For this review, take the finished solid that the model builds, in its own axes (mm). Face numbers are marked on the shaded views. A direction names the side the tool comes from. Round coordinates to 2 decimals unless told otherwise and drop trailing zeros. Loops run counter-clockwise (first coordinate to the right, second up) from the corner with the lowest first, then second, coordinate; pieces in that order, holes last.
1. To check wall thickness, follow line 1 along Z through (x, y) = (26.4, 15.24); line 2 along Z through (x, y) = (24.75, 15.5); line 3 along X through (y, z) = (25.5, -4) (3 decimals). State the ranges of each line that lie inside material, in increasing order.
2. Consider section B-B on z = -56. State the section outline as (x, y) points (3 decimals).
3. Tool access review of the marked faces 4, 5 and 6: name each direction out of +Z, -Z, +X, -X, +Y, -Y from which nothing blocks a thin tool from reaching the whole face with its end or side.
4. Consider section A-A on y = 15.24. State how many separate pieces and enclosed holes the cut face has, then the cut area to 3 significant figures.
5. Consider section D-D on z = -31.75. State the section outline as (x, y) points.
6. Clearance check with flat-ended pins moving along their axes: pin 1 Ø3 at (y, z) = (15.24, -56.42) entering from +X; pin 2 Ø3.5 at (y, z) = (12.5, -59) entering from -X; pin 3 Ø1 at (x, y) = (20.5, 20.5) entering from +Z; pin 4 Ø1.5 at (y, z) = (12.5, -16) entering from +X. State where each tip first meets the part, or that it passes through.
7. Consider section C-C on y = 18.25. State the section outline as (x, z) points (3 decimals).
8. Draft analysis for pull direction Z (two halves, no side actions). For the marked faces 1, 2 and 3, state which applies: released by +Z, released by -Z, zero draft, split by the parting line, or undercut.
from build123d import *

# Parameters (mm, degrees)
BOSS_EXTRUDE14_DEPTH = 2.54
BOSS_EXTRUDE15_DEPTH = 26.67
SKETCH5_R            = 1.905
CUT_EXTRUDE12_DEPTH  = 29.575
FILLET3_R            = 2.54


with BuildPart() as part:
    # Sketch3 → Boss-Extrude14 (new body)
    with BuildSketch(Plane(origin=(0, 0, 0), x_dir=(1, 0, 0), z_dir=(0, 1, 0))):
        with BuildLine():
            Line((0, 63.5), (0, 0))
            Line((0, 0), (24.257, 0))
            Line((24.257, 0), (24.257, 10.953386454))
            ThreePointArc((24.257, 10.953386454), (7.334843244, 31.75), (24.257, 52.546613546))
            Line((24.257, 52.546613546), (24.257, 63.5))
            Line((24.257, 63.5), (0, 63.5))
        make_face()
    extrude(amount=BOSS_EXTRUDE14_DEPTH)

    # Sketch3<18> → Boss-Extrude15 (add)
    with BuildSketch(Plane(origin=(0, 0, 0), x_dir=(1, 0, 0), z_dir=(0, 1, 0))):
        with BuildLine():
            Line((24.257, 10.953386454), (24.257, 0))
            Line((24.257, 0), (28.575, 0))
            Line((28.575, 0), (28.575, 13.081))
            ThreePointArc((28.575, 13.081), (9.906, 31.75), (28.575, 50.419))
            Line((28.575, 50.419), (28.575, 63.5))
            Line((28.575, 63.5), (24.257, 63.5))
            Line((24.257, 63.5), (24.257, 52.546613546))
            ThreePointArc((24.257, 52.546613546), (7.334843244, 31.75), (24.257, 10.953386454))
        make_face()
    extrude(amount=BOSS_EXTRUDE15_DEPTH)

    # Sketch5 → Cut-Extrude12 (cut, through all)
    with BuildSketch(Plane(origin=(0, 0, 0), x_dir=(0, 0, -1), z_dir=(1, 0, 0))):
        with Locations((6.5405, 15.24)):
            Circle(SKETCH5_R)
        with Locations((56.41762459, 15.24)):
            Circle(SKETCH5_R)
    extrude(amount=CUT_EXTRUDE12_DEPTH, mode=Mode.SUBTRACT)

    # Fillet3
    fillet3_edges = [part.edges().sort_by_distance(p)[0] for p in [
        (24.257, 2.54, -58.023306773),
        (24.257, 2.54, -5.476693227),
        (7.334843244, 2.54, -31.75),
    ]]
    fillet(fillet3_edges, radius=FILLET3_R)


solid = part.part
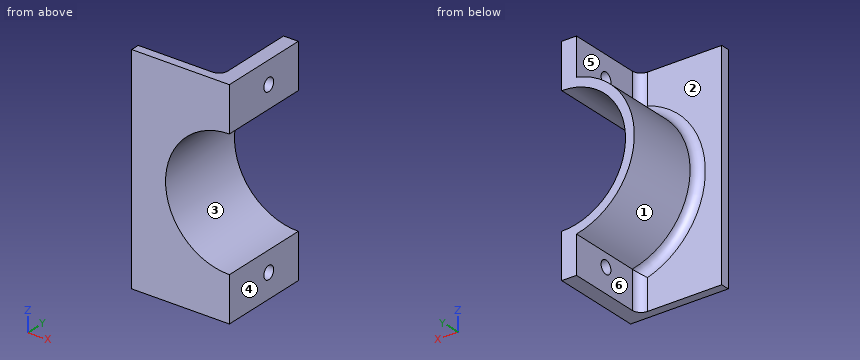
Resolved:
1. line 1: z = -63.5 to -58.32, -54.51 to -50.29, -13.21 to -8.45, -4.64 to 0
1. line 2: z = -63.5 to -58.3, -54.53 to -50.02, -13.48 to -8.43, -4.65 to 0
1. line 3: x = 24.257 to 28.575
2. outline: (0, 0) - (28.575, 0) - (28.575, 13.381) - (24.257, 13.381) - (24.257, 5.08) arc R2.54 cw to (21.717, 2.54) - (0, 2.54) - close; (24.257, 17.099) - (28.575, 17.099) - (28.575, 26.67) - (24.257, 26.67) - close
3. face 4: +Z, -Z, +X, +Y, -Y
3. face 5: +Z, -X, +Y
3. face 6: -Z, -X, +Y
4. separate pieces: 3
4. enclosed holes: 0
4. area: 220 mm2
5. outline: (0, 0) - (9.91, 0) - (9.91, 26.67) - (7.33, 26.67) - (7.33, 5.08) arc R2.54 cw to (4.79, 2.54) - (0, 2.54) - close
6. pin 1: passes through
6. pin 2: stops at x = 24.26
6. pin 3: stops at z = -11.91
6. pin 4: stops at x = 19.84
7. outline: (24.257, -63.5) - (28.575, -63.5) - (28.575, -50.419) arc R18.669 cw to (28.575, -13.081) - (28.575, 0) - (24.257, 0) - (24.257, -10.953) arc R21.24 ccw to (24.257, -52.547) - close
8. face 1: split by the parting line
8. face 2: zero draft
8. face 3: undercut
